Input: dimensioned drawing with shaded views. Units: mm. Origin: part minimum x, y, z. A direction names the side the tool comes from. Round coordinates to 2 decimals unless told otherwise and drop trailing zeros. Write each loop counter-clockwise with the first axis right and the second up, starting at its lowest first coordinate (ties: lowest second). Pieces come first, ordered by that corner, then holes. Notation, with made-up numbers: (-26, 7.5) -> (-5, 7.5) arc R26 ccw to (-5, 40.5) -> close; hole circle Ø11 at (35, -24.75). An arc over 180 degrees is marked (long way). One line per item, written item: value. Start each with the question number.
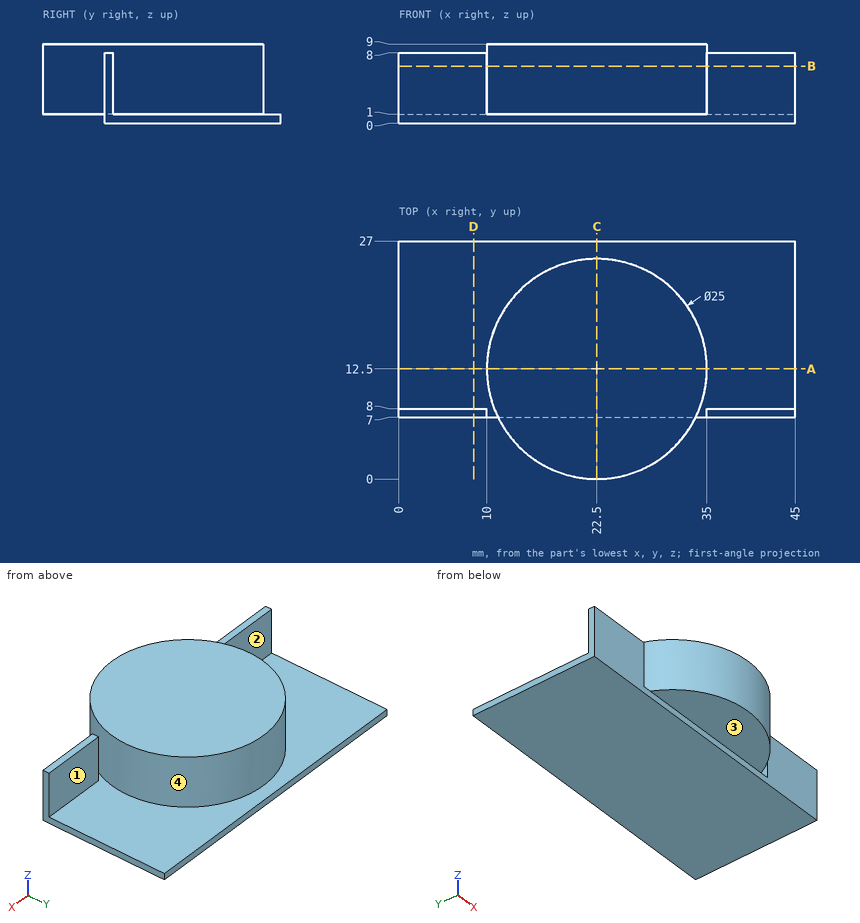
(1) Section query A-A (y = 12.5). Output: boundary loops of the cut face in (x, z).
(2) Line query: probe 1 along Y at (x, z) = (43, 7.25); probe 2 along Z at (x, y) = (25.5, 4.75); probe 3 along Z at (x, y) = (32.5, 26). Output: solid intervals per line, ascending.
(3) Set-up query: the marked faces 1, 2, 3 and 4. Return all of +Z, -Z, +X, -X, +Y, -Y with unobstructed straight access to the full face (end or side cutting, diameter ignored); none if empty.
(4) Section query D-D (x = 8.5). Output: boundary loops of the cut face in (y, z), and give its area (3 significant figures).
(5) Section query B-B (z = 6.5). Output: boundary loops of the cut face in (x, y), and give its area (3 significant figures).
(6) Pin query (flat end, axial travel): pin 1 (1.5 mm diameter, centred on y = 15, z = 8, fed in from -X); pin 2 (1 mm diameter, centred on x = 25, z = 5.5, fed in from +Y); pin 3 (2.5 mm diameter, centred on x = 29.5, z = 4.5, fed in from -Y). Return the tip coordinate at first contact, or that it passes through.
(7) Section query C-C (x = 22.5). Output: boundary loops of the cut face in (y, z), and give its area (3 significant figures).
Results list:
1. outline: (0, 0) -> (45, 0) -> (45, 1) -> (35, 1) -> (35, 9) -> (10, 9) -> (10, 1) -> (0, 1) -> close
2. probe 1: y = 7 to 8
2. probe 2: z = 1 to 9
2. probe 3: z = 0 to 1
3. face 1: +Z, +X, +Y
3. face 2: +Z, -X, +Y
3. face 3: -Z, +X, -X, -Y
3. face 4: +Z
4. outline: (7, 0) -> (27, 0) -> (27, 1) -> (8, 1) -> (8, 8) -> (7, 8) -> close
4. area: 27.0 mm^2
5. outline: (0, 7) -> (10, 7) -> (10, 8) -> (0, 8) -> close; circle Ø25 at (22.5, 12.5); (35, 7) -> (45, 7) -> (45, 8) -> (35, 8) -> close
5. area: 511 mm^2
6. pin 1: stops at x = 10.12
6. pin 2: stops at y = 24.84
6. pin 3: stops at y = 1.4
7. outline: (0, 1) -> (7, 1) -> (7, 0) -> (27, 0) -> (27, 1) -> (25, 1) -> (25, 9) -> (0, 9) -> close
7. area: 220 mm^2
